```python
from build123d import *

# Parameters (mm, degrees)
SKETCH1_W           = 60
SKETCH1_H           = 5
SKETCH1_R           = 10
SKETCH1_R_2         = 5
BOSS_EXTRUDE1_DEPTH = 5
SKETCH2_W           = 11
SKETCH2_H           = 13
SKETCH2_W_2         = 7
SKETCH2_H_2         = 7
BOSS_EXTRUDE2_DEPTH = 10
FILLET1_R           = 1


with BuildPart() as part:
    # Sketch1 → Boss-Extrude1 (new body, symmetric)
    with BuildSketch(Plane.XY):
        with BuildLine():
            Line((-50, 80.817230765), (-50, 0))
            ThreePointArc((-50, 0), (-40, 10), (-30, 0))
            Line((-30, 0), (-30, 75.817230765))
            Line((-30, 75.817230765), (-30, 80.817230765))
            Line((-30, 80.817230765), (-50, 80.817230765))
        make_face()
        with Locations((0, 78.317230765)):
            Rectangle(SKETCH1_W, SKETCH1_H)
        with BuildLine():
            Line((50, 80.817230765), (30, 80.817230765))
            Line((30, 80.817230765), (30, 75.817230765))
            Line((30, 75.817230765), (30, 0))
            ThreePointArc((30, 0), (40, 10), (50, 0))
            Line((50, 0), (50, 80.817230765))
        make_face()
        with Locations((-40, 0)):
            Circle(SKETCH1_R)
        with Locations((-40, 0)):
            Circle(SKETCH1_R_2, mode=Mode.SUBTRACT)
        with Locations((40, 0)):
            Circle(SKETCH1_R)
        with Locations((40, 0)):
            Circle(SKETCH1_R_2, mode=Mode.SUBTRACT)
    extrude(amount=BOSS_EXTRUDE1_DEPTH, both=True)

    # Sketch2 → Boss-Extrude2 (add)
    with BuildSketch(Plane.XY.offset(5)):
        with Locations((0, 69.317230765)):
            Rectangle(SKETCH2_W, SKETCH2_H)
        with Locations((0, 68.317230765)):
            Rectangle(SKETCH2_W_2, SKETCH2_H_2, mode=Mode.SUBTRACT)
    extrude(amount=-BOSS_EXTRUDE2_DEPTH)

    # Fillet1
    fillet1_edges = [part.edges().sort_by_distance(p)[0] for p in [
        (5.5, 62.817230765, 0),
        (-5.5, 62.817230765, 0),
        (-5.5, 75.817230765, 0),
        (5.5, 75.817230765, 0),
    ]]
    fillet(fillet1_edges, radius=FILLET1_R)


solid = part.part
```
Can you work these out from the model? Positions are in its coordinate system, mm. A direction names the side the tool comes from. Coordinates: 2 decimals unless noted, no trailing zeros. Loops run counter-clockwise (first coordinate to the right, second up) from the corner with the lowest first, then second, coordinate; pieces in that order, holes last. Notation, with made-up numbers: (33.5, 85.25) -> (72.5, 85.25) arc R36 ccw to (72.5, 120.25) -> close; hole circle Ø2 at (-15.75, -23.5). An arc over 180 degrees is marked (long way). Put each result on its own line as item: value. Start each with the question number.
Q1. Thinking about a two-plate mould opening in X: for faces 4 (the face through (50, 40, 0)), 5 (the face through (-50, 41, 0)), 6 (the face through (1, 80.817, 0)), 7 (the face through (30, 38, 0)), which applies, pulls with the +X half, pulls with the -X half, needs draft (parallel to the pull), parting line crosses it, or undercut?
Q2. I'm going to push flat-ended pins straight in: P1, Ø4.5, axis at x = 0.5, z = 0.5, coming from the -Y side; P2, Ø6, axis at x = -40, y = 0, coming from the +Z side; P3, Ø5, axis at x = 13.5, z = 0, coming from the -Y side. Where does each tip first touch, or does it pass through?
Q3. If I drill on line 1 (X direction, y = 22, z = -1.25); line 2 (Y direction, x = -40, z = 2.5); line 3 (Y direction, x = 1.5, z = -1.5), over which ranges is the centre line in solid material (lowest first)? Write a range as [from, to].
Q4. I want a section at A-A (x = -40). Write out the boundary of the cut face in (y, z).
Q5. I want a section at C-C (y = 70.5). Write out the boundary of the cut face in (x, z), plus the area to 3 significant figures.
Q6. I want a section at B-B (z = -2.25). Write out the boundary of the cut face in (x, y).
Q7. For faces 1 (the face through (3.5, 68, 0)), 2 (the face through (5.5, 69, 0)), 3 (the face through (-34, 36, 5)), which set-ups out of +Z, -Z, +X, -X, +Y, -Y let a thin tool reach every point of the face, with its end or its side?
Q8. I want a section at D-D (y = 32.5). Write out the boundary of the cut face in (x, z), plus the area to 3 significant figures.
Taken from the geometry:
1. face 4: pulls with the +X half
1. face 5: pulls with the -X half
1. face 6: needs draft
1. face 7: undercut
2. P1: stops at y = 62.82
2. P2: passes through
2. P3: stops at y = 75.82
3. line 1: x = [-50, -30], [30, 50]
3. line 2: y = [-10, -5], [5, 80.82]
3. line 3: y = [62.82, 64.82], [71.82, 80.82]
4. outline: (-10, -5) -> (-5, -5) -> (-5, 5) -> (-10, 5) -> close; (5, -5) -> (80.82, -5) -> (80.82, 5) -> (5, 5) -> close
5. outline: (-50, -5) -> (-30, -5) -> (-30, 5) -> (-50, 5) -> close; (-5.5, -5) -> (-3.5, -5) -> (-3.5, 5) -> (-5.5, 5) -> close; (3.5, -5) -> (5.5, -5) -> (5.5, 5) -> (3.5, 5) -> close; (30, -5) -> (50, -5) -> (50, 5) -> (30, 5) -> close
5. area: 440 mm2
6. outline: (-50, 0) arc R10 ccw to (-30, 0) -> (-30, 75.82) -> (-6.5, 75.82) arc R1 cw to (-5.5, 74.82) -> (-5.5, 63.82) arc R1 ccw to (-4.5, 62.82) -> (4.5, 62.82) arc R1 ccw to (5.5, 63.82) -> (5.5, 74.82) arc R1 cw to (6.5, 75.82) -> (30, 75.82) -> (30, 0) arc R10 ccw to (50, 0) -> (50, 80.82) -> (-50, 80.82) -> close; hole circle Ø10 at (-40, 0); hole (-3.5, 64.82) -> (3.5, 64.82) -> (3.5, 71.82) -> (-3.5, 71.82) -> close; hole circle Ø10 at (40, 0)
7. face 1: +Z, -Z
7. face 2: +Z, -Z, -Y
7. face 3: +Z, +X, -X, +Y, -Y
8. outline: (-50, -5) -> (-30, -5) -> (-30, 5) -> (-50, 5) -> close; (30, -5) -> (50, -5) -> (50, 5) -> (30, 5) -> close
8. area: 400 mm2
